```python
from build123d import *

# Parameters (mm, degrees)
EXTRUDE_1_DEPTH     = 10
EXTRUDE_2_DEPTH     = 10
SKETCH_1_8_R        = 1.35
CUT_EXTRUDE_1_DEPTH = 10
SKETCH_1_9_R        = 1.55
CUT_EXTRUDE_2_DEPTH = 10
SKETCH_1_10_R       = 9.8
CUT_EXTRUDE_3_DEPTH = 2


with BuildPart() as part:
    # Sketch 1 → Extrude 1 (new body)
    with BuildSketch(Plane.XY):
        with BuildLine():
            Line((-150, -1.5), (-150, -8.5))
            ThreePointArc((-150, -8.5), (-149.560660172, -9.560660172), (-148.5, -10))
            Line((-148.5, -10), (19.937196429, -10))
            ThreePointArc((19.937196429, -10), (29.968598214, -20.031401786), (40, -10))
            Line((40, -10), (40, -8.5))
            Line((40, -8.5), (40, 0))
            Line((40, 0), (-148.5, 0))
            ThreePointArc((-148.5, 0), (-149.560660172, -0.439339828), (-150, -1.5))
        make_face()
    extrude(amount=EXTRUDE_1_DEPTH)

    # Sketch 1_6 → Extrude 2 (add)
    with BuildSketch(Plane.XY):
        with BuildLine():
            Line((0, 0), (40, 120))
            ThreePointArc((40, 120), (64, 132), (76, 108))
            Line((76, 108), (40, 0))
            Line((40, 0), (0, 0))
        make_face()
    extrude(amount=EXTRUDE_2_DEPTH)

    # Sketch 1_8 → Cut-Extrude 1 (cut)
    with BuildSketch(Plane.XY):
        with Locations((63.349864231, 109.872544891)):
            Circle(SKETCH_1_8_R)
        with Locations((56.190864231, 117.031544891)):
            Circle(SKETCH_1_8_R)
        with Locations(Location((56.190864231, 102.713544891, 0), (0, 0, 180))):
            Circle(SKETCH_1_8_R)
        with Locations(Location((49.031864231, 109.872544891, 0), (0, 0, 180))):
            Circle(SKETCH_1_8_R)
    extrude(amount=CUT_EXTRUDE_1_DEPTH, mode=Mode.SUBTRACT)

    # Sketch 1_9 → Cut-Extrude 2 (cut)
    with BuildSketch(Plane.XY):
        with Locations((56.190864231, 109.872544891)):
            Circle(SKETCH_1_9_R)
    extrude(amount=CUT_EXTRUDE_2_DEPTH, mode=Mode.SUBTRACT)

    # Sketch 1_10 → Cut-Extrude 3 (cut)
    with BuildSketch(Plane.XY):
        with Locations((56.190864231, 109.872544891)):
            Circle(SKETCH_1_10_R)
    extrude(amount=CUT_EXTRUDE_3_DEPTH, mode=Mode.SUBTRACT)


solid = part.part
```
Check sheet for the modelled part. Datum: model origin and axes. Units: mm. A direction names the side the tool comes from. Round coordinates to 2 decimals unless told otherwise and drop trailing zeros. Order: outer loops, then holes, each group sorted by start corner. A loop starts at its lowest first (then second) coordinate and runs counter-clockwise, first axis right, second up. Notation, with made-up numbers: (84, 65) -> (129, 65) arc R19 cw to (129, 87) -> close; hole circle Ø8 at (42, -32.5). An arc over 180 degrees is marked (long way). One line per item, written item: value. Start each with the question number.
Q1. Thickness scan on line 1 (Y direction, x = -138, z = 9.75); line 2 (X direction, y = 102.5, z = 1); line 3 (X direction, y = 117, z = 3.25) (1 decimal). Record the ranges inside material, lowest first.
Q2. Set-up check for faces 4 (the face through (29.75, -20.03, 4.93)), 5 (the face through (-73, 0, 5)), 6 (the face through (40, -5, 5)), 7 (the face through (58, 110, 2)), 8 (the face through (-65, -10, 5)): record each of +Z, -Z, +X, -X, +Y, -Y from which the full face is reachable in a straight line by a thin tool's end or side.
Q3. Cross-section at B-B (x = 27). Record the boundary of the cut face in (y, z).
Q4. Cross-section at A-A (z = 6.25). Record the boundary of the cut face in (x, y), and give its area (3 significant figures).
Q5. Mould release check, pull along Y, two halves, no side actions. Record for faces 1 (the face through (48.414, 103.909, 0.986)), 2 (the face through (19.72, 59.16, 4.93)), 3 (the face through (23, 45, 10)): pulls with the +Y half, pulls with the -Y half, needs draft (parallel to the pull), parting line crosses it, or undercut.
Q6. Cross-section at C-C (y = 74). Record the boundary of the cut face in (x, z), and give its area (3 significant figures).
Q7. Gauge pin test, flat ends, axial feed: pin 1 Ø1 at (x, z) = (-11.5, 3) entering from -Y; pin 2 Ø4.5 at (x, y) = (56.19, 102.71) entering from +Z; pin 3 Ø3 at (y, z) = (-6, 5) entering from +X; pin 4 Ø1 at (x, z) = (-93, 2) entering from +Y. Record the tip position at first contact, or that the pin passes through.
Completed:
1. line 1: y = -10 to 0
1. line 2: x = 34.17 to 49.73, 62.65 to 74.17
1. line 3: x = 39 to 54.8, 57.5 to 76.7
2. face 4: +Z, -Z, -Y
2. face 5: +Z, -Z, -X, +Y
2. face 6: +Z, -Z, +X, -Y
2. face 7: -Z
2. face 8: +Z, -Z, -X, -Y
3. outline: (-19.58, 0) -> (81, 0) -> (81, 10) -> (-19.58, 10) -> close
4. outline: (-150, -8.5) arc R1.5 ccw to (-148.5, -10) -> (19.94, -10) arc R10.03 ccw to (40, -10) -> (40, 0) -> (76, 108) arc R18.97 ccw to (40, 120) -> (0, 0) -> (-148.5, 0) arc R1.5 ccw to (-150, -1.5) -> close; hole circle Ø2.7 at (49.03, 109.87); hole circle Ø3.1 at (56.19, 109.87); hole circle Ø2.7 at (56.19, 102.71); hole circle Ø2.7 at (56.19, 117.03); hole circle Ø2.7 at (63.35, 109.87)
4. area: 7,150 mm²
5. face 1: undercut
5. face 2: pulls with the +Y half
5. face 3: needs draft
6. outline: (24.67, 0) -> (64.67, 0) -> (64.67, 10) -> (24.67, 10) -> close
6. area: 400 mm²
7. pin 1: stops at y = -10
7. pin 2: stops at z = 10
7. pin 3: stops at x = 40
7. pin 4: stops at y = 0
